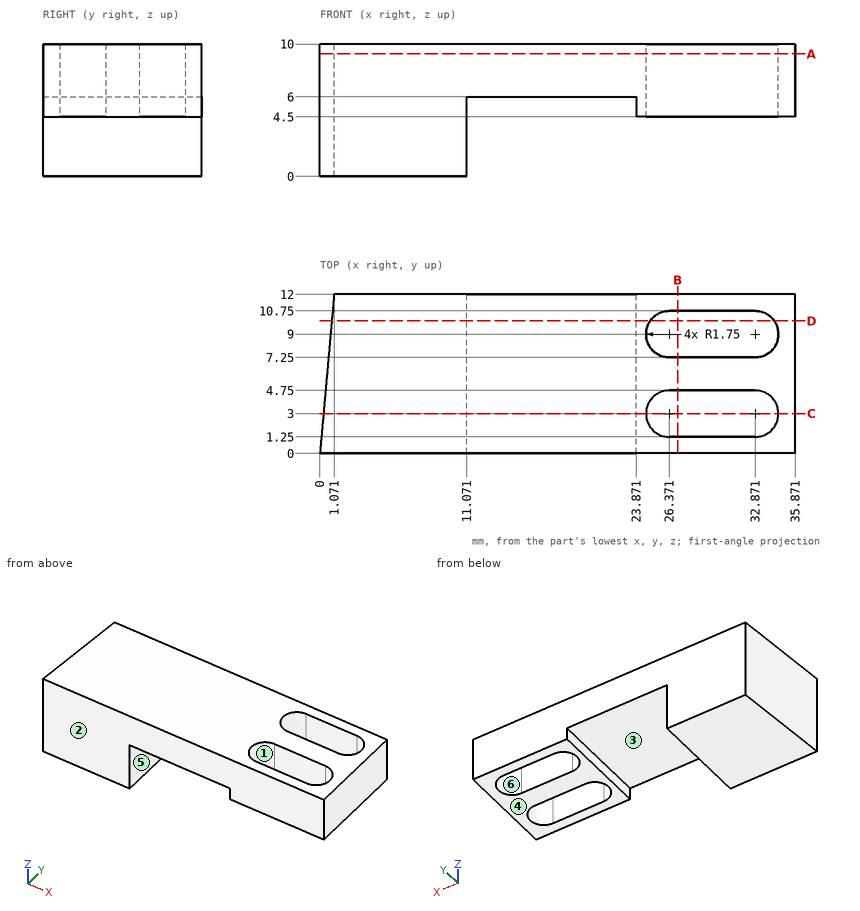
Study the drawing (mm; zero at the part's minimum x, y, z) and answer. A direction names the side the tool comes from. Give positions to 0.01 mm unless a question says otherwise; leave off trailing zeros. Write each loop counter-clockwise with the first axis right and the second up, starting at its lowest first coordinate (ties: lowest second). Pieces come first, ordered by that corner, then holes. Notation, with made-up numbers: (20, 77.25) -> (36, 77.25) arc R31 ccw to (36, 101.25) -> close; hole circle Ø1 at (27, 64). An arc over 180 degrees is marked (long way). Answer as a JSON object with one key per item and string values. Group by question number.
1) Each of these flat-tipped pins is pushed along its axis until it touches: P1, Ø0.8, axis at y = 7, z = 5, coming from the -X side; P2, Ø3.5, axis at x = 19, y = 4.5, coming from the -Z side; P3, Ø2, axis at y = 8.5, z = 8, coming from the -X side. Where does it stop, or does it pass through?
2) The mould has two halves that part along Y. Classify the marked faces 1, 2 and 3: +Y half, -Y half, draft (parallel to the pull), parting line (faces both ways), or undercut.
3) Find section B-B (x = 27). Write down the section's boundary in (y, z), and give its area (3 significant figures).
4) Find section A-A (z = 9.25). Write down the section's boundary in (x, y), and give its area (3 significant figures).
5) A tool of negligible diameter and unlimited length cuts with its end or side. For the marked faces 4, 5 and 6, from which of +Z, -Z, +X, -X, +Y, -Y can it reach the whole face along a straight path? Write none if from no direction.
6) Find section C-C (y = 3). Write down the section's boundary in (x, z).
7) Find section D-D (y = 10). Write down the section's boundary in (x, z).
8) Consider L1, parallel to X at y = 7.5, z = 5.5; L2, parallel to Y at x = 26, z = 9.5; L3, parallel to X at y = 1.75, z = 5.25. Determine where each line is inside the solid, lowest interval first. Write a range as from..to.
Values follow:
{
 "1": {"P1": "stops at x = 0.59", "P2": "stops at z = 6", "P3": "stops at x = 0.67"},
 "2": {"face 1": "undercut", "face 2": "-Y half", "face 3": "draft"},
 "3": {"outline": "(0, 4.5) -> (1.25, 4.5) -> (1.25, 10) -> (0, 10) -> close; (4.75, 4.5) -> (7.25, 4.5) -> (7.25, 10) -> (4.75, 10) -> close; (10.75, 4.5) -> (12, 4.5) -> (12, 10) -> (10.75, 10) -> close", "area": "27.5 mm2"},
 "4": {"outline": "(0, 0) -> (35.87, 0) -> (35.87, 12) -> (1.07, 12) -> close; hole (26.37, 1.25) -> (32.87, 1.25) arc R1.75 ccw to (32.87, 4.75) -> (26.37, 4.75) arc R1.75 ccw to start; hole (26.37, 7.25) -> (32.87, 7.25) arc R1.75 ccw to (32.87, 10.75) -> (26.37, 10.75) arc R1.75 ccw to start", "area": "359 mm2"},
 "5": {"face 4": "-Z, +X, +Y, -Y", "face 5": "-Z, +Y, -Y", "face 6": "+Z, -Z"},
 "6": {"outline": "(0.27, 0) -> (11.07, 0) -> (11.07, 6) -> (23.87, 6) -> (23.87, 4.5) -> (24.62, 4.5) -> (24.62, 10) -> (0.27, 10) -> close; (34.62, 4.5) -> (35.87, 4.5) -> (35.87, 10) -> (34.62, 10) -> close"},
 "7": {"outline": "(0.89, 0) -> (11.07, 0) -> (11.07, 6) -> (23.87, 6) -> (23.87, 4.5) -> (24.93, 4.5) -> (24.93, 10) -> (0.89, 10) -> close; (34.31, 4.5) -> (35.87, 4.5) -> (35.87, 10) -> (34.31, 10) -> close"},
 "8": {"L1": "x = 0.67..11.07, 23.87..25.47, 33.77..35.87", "L2": "y = 0..1.29, 4.71..7.29, 10.71..12", "L3": "x = 0.16..11.07, 23.87..25.15, 34.1..35.87"}
}
